Check sheet for the modelled part. Datum: model origin and axes. Units: mm. A direction names the side the tool comes from. Give positions to 0.01 mm unless a question says otherwise; leave off trailing zeros. Order: outer loops, then holes, each group sorted by start corner. A loop starts at its lowest first (then second) coordinate and runs counter-clockwise, first axis right, second up.
```python
from build123d import *

# Parameters (mm, degrees)
SKETCH1_R                                    = 40.5
BOSS_EXTRUDE1_DEPTH                          = 25
SHELL1_T                                     = -1
FILLET1_R                                    = 1.5
SKETCH2_W                                    = 2
SKETCH2_H                                    = 1.5
ARMCUTSMAIN_START                            = -2.5
ARMCUTSMAIN_DEPTH                            = 2.5
ARMCUTDETAIL_DEPTH                           = 5
ARMCUTDUPES_AT_THE_SECOND_PLANE_COPY_1_DEPTH = 5
HOOKS_DEPTH                                  = 2.5


with BuildPart() as part:
    # Sketch1 → Boss-Extrude1 (new body)
    with BuildSketch(Plane(origin=(0, 0, 0), x_dir=(1, 0, 0), z_dir=(0, 1, 0))):
        with BuildLine():
            Line((-23.165313871, 46), (23.165313871, 46))
            ThreePointArc((23.165313871, 46), (28.82343067, 48.001020483), (31.965545779, 53.114285714))
            ThreePointArc((31.965545779, 53.114285714), (90.537768984, 84.435627435), (111.718349922, 21.482352941))
            ThreePointArc((111.718349922, 21.482352941), (105.725511342, 0), (111.718349922, -21.482352941))
            ThreePointArc((111.718349922, -21.482352941), (90.537768984, -84.435627435), (31.965545779, -53.114285714))
            ThreePointArc((31.965545779, -53.114285714), (28.82343067, -48.001020483), (23.165313871, -46))
            Line((23.165313871, -46), (-23.165313871, -46))
            ThreePointArc((-23.165313871, -46), (-28.82343067, -48.001020483), (-31.965545779, -53.114285714))
            ThreePointArc((-31.965545779, -53.114285714), (-90.537768984, -84.435627435), (-111.718349922, -21.482352941))
            ThreePointArc((-111.718349922, -21.482352941), (-105.725511342, 0), (-111.718349922, 21.482352941))
            ThreePointArc((-111.718349922, 21.482352941), (-90.537768984, 84.435627435), (-31.965545779, 53.114285714))
            ThreePointArc((-31.965545779, 53.114285714), (-28.82343067, 48.001020483), (-23.165313871, 46))
        make_face()
        with Locations(Location((74.5, 44, 0), (0, 0, 270))):
            Circle(SKETCH1_R, mode=Mode.SUBTRACT)
        with Locations(Location((74.5, -44, 0), (0, 0, 90))):
            Circle(SKETCH1_R, mode=Mode.SUBTRACT)
        with Locations(Location((-74.5, -44, 0), (0, 0, 270))):
            Circle(SKETCH1_R, mode=Mode.SUBTRACT)
        with Locations(Location((-74.5, 44, 0), (0, 0, 90))):
            Circle(SKETCH1_R, mode=Mode.SUBTRACT)
    extrude(amount=BOSS_EXTRUDE1_DEPTH)

    # Shell1
    shell1_openings = [part.faces().sort_by_distance(p)[0] for p in [
        (0, 25, 0),
    ]]
    offset(amount=SHELL1_T, openings=shell1_openings, kind=Kind.INTERSECTION)

    # Fillet1
    fillet1_edges = [part.edges().sort_by_distance(p)[0] for p in [
        (74.5, 0, -84.5),
        (74.5, 0, 84.5),
        (-74.5, 0, 3.5),
        (-74.5, 0, -3.5),
    ]]
    fillet(fillet1_edges, radius=FILLET1_R)

    # Lip: sweep along a path in Sketch1_2
    with BuildLine(Plane(origin=(0, 0, 0), x_dir=(1, 0, 0), z_dir=(0, 1, 0))) as lip_path:
        Line((-23.165313871, 46), (23.165313871, 46))
        ThreePointArc((23.165313871, 46), (28.82343067, 48.001020483), (31.965545779, 53.114285714))
        ThreePointArc((31.965545779, 53.114285714), (90.537768984, 84.435627435), (111.718349922, 21.482352941))
        ThreePointArc((111.718349922, 21.482352941), (105.725511342, 0), (111.718349922, -21.482352941))
        ThreePointArc((111.718349922, -21.482352941), (90.537768984, -84.435627435), (31.965545779, -53.114285714))
        ThreePointArc((31.965545779, -53.114285714), (28.82343067, -48.001020483), (23.165313871, -46))
        Line((23.165313871, -46), (-23.165313871, -46))
        ThreePointArc((-23.165313871, -46), (-28.82343067, -48.001020483), (-31.965545779, -53.114285714))
        ThreePointArc((-31.965545779, -53.114285714), (-90.537768984, -84.435627435), (-111.718349922, -21.482352941))
        ThreePointArc((-111.718349922, -21.482352941), (-105.725511342, 0), (-111.718349922, 21.482352941))
        ThreePointArc((-111.718349922, 21.482352941), (-90.537768984, 84.435627435), (-31.965545779, 53.114285714))
        ThreePointArc((-31.965545779, 53.114285714), (-28.82343067, 48.001020483), (-23.165313871, 46))
    # Sketch2 → Lip (sweep)
    with BuildSketch(Plane(origin=(0, 0, 0), x_dir=(0, 0, -1), z_dir=(1, 0, 0))):
        with Locations((-47, 0.75)):
            Rectangle(SKETCH2_W, SKETCH2_H)
    sweep(path=lip_path.line)

    # Sketch3 → ArmCutsMain (cut)
    with BuildSketch(Plane(origin=(0, 25, 0), x_dir=(1, 0, 0), z_dir=(0, 1, 0)).offset(ARMCUTSMAIN_START)):
        with BuildLine():
            ThreePointArc((-34.813352628, -31.866574254), (-33.45584167, -37.865909438), (-33, -44))
            Line((-33, -44), (-74.5, -44))
            Line((-74.5, -44), (-34.813352628, -31.866574254))
        make_face()
        with BuildLine():
            Line((74.5, -44), (34.813352628, -31.866574254))
            ThreePointArc((34.813352628, -31.866574254), (33.45584167, -37.865909438), (33, -44))
            Line((33, -44), (74.5, -44))
        make_face()
        with BuildLine():
            Line((-74.5, 44), (-34.813352628, 31.866574254))
            ThreePointArc((-34.813352628, 31.866574254), (-33.45584167, 37.865909438), (-33, 44))
            Line((-33, 44), (-74.5, 44))
        make_face()
        with BuildLine():
            ThreePointArc((34.813352628, 31.866574254), (33.45584167, 37.865909438), (33, 44))
            Line((33, 44), (74.5, 44))
            Line((74.5, 44), (34.813352628, 31.866574254))
        make_face()
    extrude(amount=ARMCUTSMAIN_DEPTH, mode=Mode.SUBTRACT)

    # Sketch6 → ArmCutDetail (cut)
    with BuildSketch(Plane(origin=(39.689358355, 0, 5.931614349), x_dir=(-0.14780941112961088, 0, 0.9890158633619168), z_dir=(-0.9890158633619167, 0, -0.14780941112961085))):
        with BuildLine():
            Line((34.518615708, 22.5), (30.518615708, 22.5))
            Line((30.518615708, 22.5), (30.518615708, 22.1))
            ThreePointArc((30.518615708, 22.1), (30.694351639, 21.675735931), (31.118615708, 21.5))
            Line((31.118615708, 21.5), (33.918615708, 21.5))
            ThreePointArc((33.918615708, 21.5), (34.342879777, 21.675735931), (34.518615708, 22.1))
            Line((34.518615708, 22.1), (34.518615708, 22.5))
        make_face()
    armcutdetail = extrude(amount=ARMCUTDETAIL_DEPTH, mode=Mode.SUBTRACT)

    # ArmCutDupes: ArmCutDetail across plane
    add(armcutdetail.mirror(Plane(origin=(0, 0, 0), x_dir=(0, 0, 1), z_dir=(1, 0, 0))), mode=Mode.SUBTRACT)

    # ArmCutDupes at the second plane: ArmCutDetail across plane
    add(armcutdetail.mirror(Plane.XY), mode=Mode.SUBTRACT)

    # ArmCutDupes at the second plane copy 1 s → ArmCutDupes at the second plane copy 1 (cut)
    with BuildSketch(Plane(origin=(-39.689358355, 0, -5.931614349), x_dir=(0.14780941112961088, 0, -0.9890158633619168), z_dir=(0.9890158633619167, 0, 0.14780941112961085))):
        with BuildLine():
            Line((34.518615708, 22.5), (30.518615708, 22.5))
            Line((30.518615708, 22.5), (30.518615708, 22.1))
            ThreePointArc((30.518615708, 22.1), (30.694351639, 21.675735931), (31.118615708, 21.5))
            Line((31.118615708, 21.5), (33.918615708, 21.5))
            ThreePointArc((33.918615708, 21.5), (34.342879777, 21.675735931), (34.518615708, 22.1))
            Line((34.518615708, 22.1), (34.518615708, 22.5))
        make_face()
    extrude(amount=ARMCUTDUPES_AT_THE_SECOND_PLANE_COPY_1_DEPTH, mode=Mode.SUBTRACT)

    # Sketch7 → Hooks (add, symmetric)
    with BuildSketch(Plane(origin=(0, 0, 0), x_dir=(0, 0, -1), z_dir=(1, 0, 0))):
        Polygon((46, 25), (49.5, 25), (49.5, 22), (48.25, 22), (48.25, 23.5), (46, 23.5), align=None)
        Polygon((-46, 23.5), (-46, 25), (-49.5, 25), (-49.5, 22), (-48.25, 22), (-48.25, 23.5), align=None)
    extrude(amount=HOOKS_DEPTH, both=True)


solid = part.part
```
(1) Cross-section at A-A on x = -74.5. Count the separate pieces of the cut face and the enclosed holes in it, then the cut area to 3 significant figures.
Response values:
separate pieces: 3
enclosed holes: 0
area: 161 mm2
(2) Cross-section at C-C on x = 0. Enter the section's corners in (y, z), then the cut area to 3 significant figures.
Response values:
outline: (0, -48) - (1.5, -48) - (1.5, -46) - (23.5, -46) - (23.5, -48.25) - (22, -48.25) - (22, -49.5) - (25, -49.5) - (25, -45) - (1, -45) - (1, 45) - (25, 45) - (25, 49.5) - (22, 49.5) - (22, 48.25) - (23.5, 48.25) - (23.5, 46) - (1.5, 46) - (1.5, 48) - (0, 48) - close
area: 160 mm2
(3) Material ranges on L1, parallel to X at y = 16.5, z = 44; L2, parallel to Z at x = -53, y = 15; L3, parallel to X at y = 2.25, z = 14, recorded low to high.
Response values:
L1: x = -118 to -117, -116 to -115, -34 to -33, 33 to 34, 115 to 116, 117 to 118
L2: z = -81.82 to -80.66, -79.5 to -78.32, -9.68 to -8.5, 8.5 to 9.68, 78.32 to 79.5, 80.66 to 81.82
L3: x = -108.16 to -107.1, -103.17 to -101.71, -47.29 to -45.83, 45.83 to 47.29, 101.71 to 103.17, 107.1 to 108.16
(4) Set-up check for faces 4 (the face through (107.727, 0.74, -0.301)), 5 (the face through (105.727, 13.086, -0.316)), 6 (the face through (1, 1, 0)): record each of +Z, -Z, +X, -X, +Y, -Y from which the full face is reachable in a straight line by a thin tool's end or side.
Response values:
face 4: +X, +Y, -Y
face 5: +X, +Y
face 6: +Y
(5) Gauge pin test, flat ends, axial feed: pin 1 Ø1 at (y, z) = (8, -39.5) entering from -X; pin 2 Ø4 at (y, z) = (15, -18) entering from +X; pin 3 Ø0.6 at (x, z) = (34.5, -34.5) entering from +Y. Record the tip position at first contact, or that the pin passes through.
Response values:
pin 1: stops at x = -117.82
pin 2: stops at x = 110.86
pin 3: stops at y = 22.5
(6) Release check for a two-part mould opening along Z. For faces 1 (the face through (27.51, 0.74, -49.51)), 2 (the face through (-27.51, 0.74, 49.51)), 3 (the face through (-108.65, 13.09, -65.77)) record: released by +Z, released by -Z, zero draft, split by the parting line, or undercut.
Response values:
face 1: released by -Z
face 2: released by +Z
face 3: undercut
